from build123d import *

# Parameters (mm, degrees)
BASEPIEDEAPPOGGIO_START = -10.5
BASEPIEDEAPPOGGIO_DEPTH = 21
LATOSINISTRO_DEPTH      = 2
SCHIZZO3_W              = 5
SCHIZZO3_H              = 3
ALETTEAGGANCIO_DEPTH    = 30


# Read off the part's stored shape, not the designer's step: BasePiedeAppoggio
with BuildPart() as part:
    # BasePiedeAppoggio outline → BasePiedeAppoggio (new body)
    with BuildSketch(Plane(origin=(0, 0, 0), x_dir=(0, 0, -1), z_dir=(1, 0, 0)).offset(BASEPIEDEAPPOGGIO_START)):
        with BuildLine():
            Line((-67, -6.58541733), (-67, -7.5))
            add(Edge.make_bspline(
                [(-67, -7.5), (-60, -14), (-44, -17), (-14, -13), (-5, -8), (0, 0)],
                knots=[0, 0, 0, 0, 0, 0, 1, 1, 1, 1, 1, 1], degree=5))
            Line((0, 0), (0, 2))
            Line((0, 2), (-2.409917527, 2))
            Line((-2.409917527, 2), (-2.409917527, 0))
            add(Edge.make_bspline(
                [(-2.409917527, 0), (-2.667324323, -0.353402954), (-3.476108464, -1.377540434), (-5.718312008, -3.574118885), (-10.497685703, -6.435761001), (-19.037438877, -9.233820798), (-29.572047533, -11.136431528), (-38.966676556, -11.799385995), (-46.135832891, -11.693755764), (-51.166703498, -11.28631183), (-55.693282116, -10.549034431), (-58.932001396, -9.671882802), (-61.157085706, -8.829738395), (-62.633910182, -8.137838289), (-63.931461685, -7.382278902), (-64.645771008, -6.869387628), (-65, -6.58541733)],
                knots=[0.030225408, 0.030225408, 0.030225408, 0.030225408, 0.061229523, 0.122459046, 0.244918093, 0.367377139, 0.489836186, 0.612295232, 0.673524756, 0.734754279, 0.795983802, 0.857213325, 0.887828087, 0.918442849, 0.94905761, 0.979672372, 0.979672372, 0.979672372, 0.979672372], degree=3))
            Line((-65, -6.58541733), (-67, -6.58541733))
        make_face()
    extrude(amount=BASEPIEDEAPPOGGIO_DEPTH)

    # Schizzo2 → LatoSinistro (add)
    with BuildSketch(Plane.ZY.offset(10.5)):
        with BuildLine():
            Line((67, -7.5), (67, 2))
            Line((67, 2), (0, 2))
            Line((0, 2), (0, 0))
            add(Edge.make_bspline(
                [(67, -7.5), (60, -14), (44, -17), (14, -13), (5, -8), (0, 0)],
                knots=[0, 0, 0, 0, 0, 0, 1, 1, 1, 1, 1, 1], degree=5))
        make_face()
    latosinistro = extrude(amount=-LATOSINISTRO_DEPTH)

    # LatoDestro: LatoSinistro across plane
    add(latosinistro.mirror(Plane(origin=(0, 0, 0), x_dir=(0, 0, 1), z_dir=(1, 0, 0))))

    # Schizzo3 → AletteAggancio (add)
    with BuildSketch(Plane.XY.offset(67)):
        with Locations((-13, 0.5)):
            Rectangle(SCHIZZO3_W, SCHIZZO3_H)
        with Locations((13, 0.5)):
            Rectangle(SCHIZZO3_W, SCHIZZO3_H)
    extrude(amount=-ALETTEAGGANCIO_DEPTH)


solid = part.part
Could you check a few things on this model? Use its own coordinates, in mm. A direction names the side the tool comes from. Round coordinates to 2 decimals unless told otherwise and drop trailing zeros. Order: outer loops, then holes, each group sorted by start corner. A loop starts at its lowest first (then second) coordinate and runs counter-clockwise, first axis right, second up.
(1) I'm going to push flat-ended pins straight in: pin 1 (10 mm diameter, centred on x = -5.5, z = 50.5, fed in from -Y); pin 2 (1 mm diameter, centred on x = -3.5, z = 66, fed in from +Y); pin 3 (0.9 mm diameter, centred on x = -12, y = 1, fed in from -Z); pin 4 (10 mm diameter, centred on x = 7.5, z = 40, fed in from +Y). Where does each tip first touch, or does it pass through?
Response values:
pin 1: stops at y = -13.67
pin 2: stops at y = -6.59
pin 3: stops at z = 37
pin 4: stops at y = 2
(2) Please list where these lines run through material, in increasing order: line 1 along X through (y, z) = (1.75, 43); line 2 along X through (y, z) = (-3.75, 14.5); line 3 along X through (y, z) = (-9.25, 18.5).
Response values:
line 1: x = -15.5 to -8.5, 8.5 to 15.5
line 2: x = -10.5 to -8.5, 8.5 to 10.5
line 3: x = -10.5 to 10.5
(3) Which directions (+Z, -Z, +X, -X, +Y, -Y) give clear straight access to the entire face, cutting with the end or side of a thin tool? Please do faces 1 (the flat face through (8.5, -3, 34)), 2 (the flat face through (-13, -1, 52)), 3 (the flat face through (13, 1, 37)), 4 (the flat face through (0, 1, 2.41)).
Response values:
face 1: +Y
face 2: +Z, -Z, -X, -Y
face 3: -Z, +X, +Y, -Y
face 4: +Z, +Y
(4) Imagine slicing it at A-A (x = 13.5). Write out the boundary of the cut face in (y, z), plus the area to 3 significant figures.
Response values:
outline: (-1, 37) - (2, 37) - (2, 67) - (-1, 67) - close
area: 90.0 mm2
(5) If we mould it in two halves opening along X, with no side actions, what happens to faces 5 (the flat face through (13, -1, 52)), 6 (the flat face through (15.5, 0, 52)), 7 (the flat face through (-8.5, -3, 34))? For each: released by +X, released by -X, zero draft, split by the parting line, or undercut.
Response values:
face 5: zero draft
face 6: released by +X
face 7: undercut
